Input: part model. Units: mm. Frame: model coordinates. A direction names the side the tool comes from. Round coordinates to 2 decimals unless told otherwise and drop trailing zeros. Write each loop counter-clockwise with the first axis right and the second up, starting at its lowest first coordinate (ties: lowest second). Pieces come first, ordered by that corner, then holes. Notation, with made-up numbers: M 63.25,5 L 81.25,5 A9 ccw 81.25,15 Z; hole C -2,19 d7. An arc over 180 degrees is marked long. Use one line per item in the form item = value. Start each with the question number.
```python
from build123d import *

# Parameters (mm, degrees)
PAD_DEPTH    = 6.15
POCKET_DEPTH = 3
PAD001_DEPTH = 4
CHAMFER_SIZE = 0.2


with BuildPart() as part:
    # Sketch → Pad (new body)
    with BuildSketch(Plane.XY):
        with BuildLine():
            Line((-9, 7.5), (-9, -7.5))
            ThreePointArc((-9, -7.5), (-8.56066, -8.56066), (-7.5, -9))
            Line((-7.5, -9), (7.5, -9))
            ThreePointArc((7.5, -9), (8.56066, -8.56066), (9, -7.5))
            Line((9, -7.5), (9, 7.5))
            ThreePointArc((9, 7.5), (8.56066, 8.56066), (7.5, 9))
            Line((7.5, 9), (-7.5, 9))
            ThreePointArc((-7.5, 9), (-8.56066, 8.56066), (-9, 7.5))
        make_face()
    extrude(amount=PAD_DEPTH)

    # Sketch001 (on Face9 of Pad) → Pocket (cut)
    with BuildSketch(Plane(origin=(0, 0, 0), x_dir=(1, 0, 0), z_dir=(0, 0, -1))):
        with BuildLine():
            Line((-7.8, 6.3), (-7.8, -6.3))
            ThreePointArc((-7.8, -6.3), (-7.36066, -7.36066), (-6.3, -7.8))
            Line((-6.3, -7.8), (6.3, -7.8))
            ThreePointArc((6.3, -7.8), (7.36066, -7.36066), (7.8, -6.3))
            Line((7.8, -6.3), (7.8, 6.3))
            ThreePointArc((7.8, 6.3), (7.36066, 7.36066), (6.3, 7.8))
            Line((6.3, 7.8), (-6.3, 7.8))
            ThreePointArc((-6.3, 7.8), (-7.36066, 7.36066), (-7.8, 6.3))
        make_face()
    extrude(amount=-POCKET_DEPTH, mode=Mode.SUBTRACT)

    # Sketch002 (on Face19 of Pocket) → Pad001 (join)
    with BuildSketch(Plane(origin=(0, 0, 3), x_dir=(1, 0, 0), z_dir=(0, 0, -1))):
        Polygon((-3.425, -1.45), (-2.275, -1.45), (-2.275, -0.2), (-2.175, -0.2), (-2.175, 0.2), (-2.275, 0.2), (-2.275, 1.45), (-3.425, 1.45), (-3.425, 0.2), (-3.525, 0.2), (-3.525, -0.2), (-3.425, -0.2), align=None)
        Polygon((3.425, 1.45), (2.275, 1.45), (2.275, 0.2), (2.175, 0.2), (2.175, -0.2), (2.275, -0.2), (2.275, -1.45), (3.425, -1.45), (3.425, -0.2), (3.525, -0.2), (3.525, 0.2), (3.425, 0.2), align=None)
    extrude(amount=PAD001_DEPTH)

    # Chamfer
    chamfer_edges = [part.edges().sort_by_distance(p)[0] for p in [
        (0, -9, 6.15),
    ]]
    chamfer(chamfer_edges, length=CHAMFER_SIZE)


solid = part.part
```
Item 1: First-contact query: pin 1 (2 mm diameter, centred on x = 3.5, y = -1, fed in from -Z). Flat tip, straight axial feed; report the tip coordinate or a pass-through.
Item 2: Draft query along X for faces 1 (the face through (8.55, -8.57, 2.93)), 2 (the face through (-8, 0, 0)), 3 (the face through (3.425, -1, 1)). Return one class per face: +X half, -X half, draft (parallel to the pull), parting line (faces both ways), or undercut.
Item 3: Cut plane C-C (z = 2.25). Give the number of separate pieces and of enclosed holes in the cut face, plus the area to 3 significant figures.
Item 4: Cut plane B-B (x = -5.75). Output: boundary loops of the cut face in (y, z).
Item 5: Reachability of faces 4 (the face through (-3, -1.45, 1)), 5 (the face through (3, 0, -1)) from +Z, -Z, +X, -X, +Y, -Y: full face, straight path, thin tool, end or side. Return the list, or none.
Item 6: Cut plane A-A (z = -0.5). Output: boundary loops of the cut face in (x, y) (3 decimals), plus the area to 3 significant figures.
Item 7: Ray query, line 1 (Y direction, x = 3, z = 1.5); line 2 (X direction, y = 0, z = 2.5) (3 decimals); line 3 (X direction, y = -1.25, z = 1) (3 decimals). Return the intervals inside material, ascending. Write a range as from..to.
Final values:
q1.pin_1 = -1
q2.face_1 = +X half
q2.face_2 = draft
q2.face_3 = undercut
q3.separate_pieces = 3
q3.enclosed_holes = 1
q3.area = 87.5 mm^2
q4.outline = M -9,0 L -7.8,0 L -7.8,3 L 7.8,3 L 7.8,0 L 9,0 L 9,5.95 L 8.8,6.15 L -8.8,6.15 L -9,5.95 Z
q5.face_4 = -Z
q5.face_5 = -Z, +X, -X, +Y, -Y
q6.outline = M -3.525,-0.2 L -3.425,-0.2 L -3.425,-1.45 L -2.275,-1.45 L -2.275,-0.2 L -2.175,-0.2 L -2.175,0.2 L -2.275,0.2 L -2.275,1.45 L -3.425,1.45 L -3.425,0.2 L -3.525,0.2 Z; M 2.175,-0.2 L 2.275,-0.2 L 2.275,-1.45 L 3.425,-1.45 L 3.425,-0.2 L 3.525,-0.2 L 3.525,0.2 L 3.425,0.2 L 3.425,1.45 L 2.275,1.45 L 2.275,0.2 L 2.175,0.2 Z
q6.area = 6.83 mm^2
q7.line_1 = -9..-7.8, -1.45..1.45, 7.8..9
q7.line_2 = -9..-7.8, -3.525..-2.175, 2.175..3.525, 7.8..9
q7.line_3 = -9..-7.8, -3.425..-2.275, 2.275..3.425, 7.8..9
